from build123d import *

# Parameters (mm, degrees)
F0_W          = 54
F0_H          = 54
F1_DEPTH      = 2
F2_W          = 54
F2_H          = 54
F2_W_2        = 50.3
F2_H_2        = 50.3
F3_DEPTH      = 10.2
F4_R          = 3.5
F5_DEPTH      = 5.5
F6_R          = 1.6
F7_DEPTH      = 25
F8_W          = 9.5
F8_H          = 4.75
F9_DEPTH      = 25
F11_DEPTH     = 25
F12_T1_DEPTH  = 48
F12_T3_DEPTH  = 48
F12_T5_DEPTH  = 16.7
F12_S9_W      = 3
F12_S9_H      = 3
F12_T10_DEPTH = 3
F12_S15_W     = 3
F12_S15_H     = 3
F12_T16_DEPTH = 3
F12_S21_W     = 3
F12_S21_H     = 3
F12_T22_DEPTH = 3
F12_S27_W     = 3
F12_S27_H     = 3
F12_T28_DEPTH = 3
F13_R         = 3
F14_DEPTH     = 2.5
F15_R         = 0.8
F16_R         = 2


# Not quite as in the source:
# - a fillet or chamfer that OpenCascade refuses, or shapes differently, is made with other operations: its cross-section is extruded or revolved along the edge and cut away or added


with BuildPart() as f1:
    # F0 (on Top) → F1 (new body)
    with BuildSketch(Plane.XY):
        Rectangle(F0_W, F0_H)
    extrude(amount=F1_DEPTH)

    # F2 (on face) → F3 (join)
    with BuildSketch(Plane.XY.offset(2)):
        Rectangle(F2_W, F2_H)
        Rectangle(F2_W_2, F2_H_2, mode=Mode.SUBTRACT)
    extrude(amount=F3_DEPTH)

    # F4 (on face) → F5 (join)
    with BuildSketch(Plane.XY.offset(2)):
        with Locations((-22.5, 22.5)):
            Circle(F4_R)
        with Locations((22.5, 22.5)):
            Circle(F4_R)
        with Locations((22.5, -22.5)):
            Circle(F4_R)
        with Locations((-22.5, -22.5)):
            Circle(F4_R)
    extrude(amount=F5_DEPTH)

    # F6 (on face) → F7 (cut)
    with BuildSketch(Plane(origin=(0, 0, 0), x_dir=(1, 0, 0), z_dir=(0, 0, -1))):
        with Locations((-22.5, 22.5)):
            Circle(F6_R)
        with Locations((22.5, 22.5)):
            Circle(F6_R)
        with Locations((22.5, -22.5)):
            Circle(F6_R)
        with Locations((-22.5, -22.5)):
            Circle(F6_R)
        Circle(F6_R)
    extrude(amount=-F7_DEPTH, mode=Mode.SUBTRACT)

    # F8 (on face) → F9 (cut)
    with BuildSketch(Plane.XZ.offset(27)):
        with Locations((13.25, 5.875)):
            Rectangle(F8_W, F8_H)
    extrude(amount=-F9_DEPTH, mode=Mode.SUBTRACT)

    # F10 (on face) → F11 (cut)
    with BuildSketch(Plane.XY.offset(2)):
        with BuildLine():
            add(Edge.make_bspline(
                [(-20.15, 4.5483106502), (-23.5056844979, 4.5483106502), (-21.827842249, -2.2741553251), (-20.15, -9.0966213004), (-18.472157751, -2.2741553251), (-16.7943155021, 4.5483106502), (-20.15, 4.5483106502)],
                knots=[0, 0, 0, 2.0943951024, 2.0943951024, 4.1887902048, 4.1887902048, 6.2831853072, 6.2831853072, 6.2831853072], degree=2, weights=[1, 0.5, 1, 0.5, 1, 0.5, 1]))
        make_face()
    extrude(amount=-F11_DEPTH, mode=Mode.SUBTRACT)

    # F12: fillet of radius 3 on 8 edges, made by hand

    # F12_s2 → F12_t1 (cut)
    with BuildSketch(Plane.YZ.offset(-24)):
        with BuildLine():
            ThreePointArc((-24, 0), (-26.1213203436, 0.8786796564), (-27, 3))
            Line((-27, 3), (-27, 0))
            Line((-27, 0), (-24, 0))
        make_face()
        with BuildLine():
            ThreePointArc((27, 3), (26.1213203436, 0.8786796564), (24, 0))
            Line((24, 0), (27, 0))
            Line((27, 0), (27, 3))
        make_face()
    extrude(amount=F12_T1_DEPTH, mode=Mode.SUBTRACT)

    # F12_s4 → F12_t3 (cut)
    with BuildSketch(Plane.XZ.offset(-24)):
        with BuildLine():
            ThreePointArc((-27, 3), (-26.1213203436, 0.8786796564), (-24, 0))
            Line((-24, 0), (-27, 0))
            Line((-27, 0), (-27, 3))
        make_face()
        with BuildLine():
            ThreePointArc((27, 3), (26.1213203436, 0.8786796564), (24, 0))
            Line((24, 0), (27, 0))
            Line((27, 0), (27, 3))
        make_face()
    extrude(amount=F12_T3_DEPTH, mode=Mode.SUBTRACT)

    # F12_s6 → F12_t5 (cut)
    with BuildSketch(Plane.XY.offset(3)):
        with BuildLine():
            ThreePointArc((27, -24), (26.1213203436, -26.1213203436), (24, -27))
            Line((24, -27), (27, -27))
            Line((27, -27), (27, -24))
        make_face()
        with BuildLine():
            ThreePointArc((-27, -24), (-26.1213203436, -26.1213203436), (-24, -27))
            Line((-24, -27), (-27, -27))
            Line((-27, -27), (-27, -24))
        make_face()
        with BuildLine():
            ThreePointArc((-24, 27), (-26.1213203436, 26.1213203436), (-27, 24))
            Line((-27, 24), (-27, 27))
            Line((-27, 27), (-24, 27))
        make_face()
        with BuildLine():
            ThreePointArc((24, 27), (26.1213203436, 26.1213203436), (27, 24))
            Line((27, 24), (27, 27))
            Line((27, 27), (24, 27))
        make_face()
    extrude(amount=F12_T5_DEPTH, mode=Mode.SUBTRACT)


with BuildPart() as f12_tool8:
    # F12_s9 → F12_t10 (new body)
    with BuildSketch(Plane.YZ.offset(-24)):
        with Locations((-25.5, 1.5)):
            Rectangle(F12_S9_W, F12_S9_H)
    extrude(amount=-F12_T10_DEPTH)

    # F12_s11 → F12_t12 (revolve, cut)
    with BuildSketch(Plane(origin=(-24, -24, 3), x_dir=(0, 0.7071067812, 0.7071067812), z_dir=(0, -0.7071067812, 0.7071067812))):
        with BuildLine():
            ThreePointArc((0, -3), (3, 0), (0, 3))
            Line((0, 3), (0, -3))
        make_face()
    revolve(axis=Axis((-24, -24, 3), (-1, 0, 0)), mode=Mode.SUBTRACT)


with BuildPart() as f1_1:
    add(f1.part)

    # F12_t7: cut F12_tool8
    add(f12_tool8.part, mode=Mode.SUBTRACT)


with BuildPart() as f12_tool14:
    # F12_s15 → F12_t16 (new body)
    with BuildSketch(Plane.YZ.offset(24)):
        with Locations((-25.5, 1.5)):
            Rectangle(F12_S15_W, F12_S15_H)
    extrude(amount=F12_T16_DEPTH)

    # F12_s17 → F12_t18 (revolve, cut)
    with BuildSketch(Plane(origin=(24, -24, 3), x_dir=(0, 0.7071067812, 0.7071067812), z_dir=(0, 0.7071067812, -0.7071067812))):
        with BuildLine():
            ThreePointArc((0, -3), (3, 0), (0, 3))
            Line((0, 3), (0, -3))
        make_face()
    revolve(axis=Axis((24, -24, 3), (1, 0, 0)), mode=Mode.SUBTRACT)


with BuildPart() as f1_2:
    add(f1_1.part)

    # F12_t13: cut F12_tool14
    add(f12_tool14.part, mode=Mode.SUBTRACT)


with BuildPart() as f12_tool20:
    # F12_s21 → F12_t22 (new body)
    with BuildSketch(Plane.XZ.offset(-24)):
        with Locations((-25.5, 1.5)):
            Rectangle(F12_S21_W, F12_S21_H)
    extrude(amount=-F12_T22_DEPTH)

    # F12_s23 → F12_t24 (revolve, cut)
    with BuildSketch(Plane(origin=(-24, 24, 3), x_dir=(0.7071067812, 0, 0.7071067812), z_dir=(-0.7071067812, 0, 0.7071067812))):
        with BuildLine():
            ThreePointArc((0, -3), (3, 0), (0, 3))
            Line((0, 3), (0, -3))
        make_face()
    revolve(axis=Axis((-24, 24, 3), (0, 1, 0)), mode=Mode.SUBTRACT)


with BuildPart() as f1_3:
    add(f1_2.part)

    # F12_t19: cut F12_tool20
    add(f12_tool20.part, mode=Mode.SUBTRACT)


with BuildPart() as f12_tool26:
    # F12_s27 → F12_t28 (new body)
    with BuildSketch(Plane.XZ.offset(-24)):
        with Locations((25.5, 1.5)):
            Rectangle(F12_S27_W, F12_S27_H)
    extrude(amount=-F12_T28_DEPTH)

    # F12_s29 → F12_t30 (revolve, cut)
    with BuildSketch(Plane(origin=(24, 24, 3), x_dir=(-0.7071067812, 0, 0.7071067812), z_dir=(-0.7071067812, 0, -0.7071067812))):
        with BuildLine():
            ThreePointArc((0, -3), (3, 0), (0, 3))
            Line((0, 3), (0, -3))
        make_face()
    revolve(axis=Axis((24, 24, 3), (0, 1, 0)), mode=Mode.SUBTRACT)


with BuildPart() as f1_4:
    add(f1_3.part)

    # F12_t25: cut F12_tool26
    add(f12_tool26.part, mode=Mode.SUBTRACT)

    # F13 (on face) → F14 (cut)
    with BuildSketch(Plane(origin=(0, 0, 0), x_dir=(1, 0, 0), z_dir=(0, 0, -1))):
        with Locations((-22.5, 22.5)):
            Circle(F13_R)
        with Locations((22.5, 22.5)):
            Circle(F13_R)
        with Locations((22.5, -22.5)):
            Circle(F13_R)
        with Locations((-22.5, -22.5)):
            Circle(F13_R)
    extrude(amount=-F14_DEPTH, mode=Mode.SUBTRACT)

    # F15
    f15_edges = [f1_4.edges().sort_by_distance(p)[0] for p in [
        (8.5, -26.075, 8.25),
        (8.5, -26.075, 3.5),
        (18, -26.075, 3.5),
        (18, -26.075, 8.25),
    ]]
    fillet(f15_edges, radius=F15_R)

    # F16
    f16_edges = [f1_4.edges().sort_by_distance(p)[0] for p in [
        (-25.15, 25.15, 7.1),
        (25.15, 25.15, 7.1),
        (-25.15, -25.15, 7.1),
        (25.15, -25.15, 7.1),
    ]]
    fillet(f16_edges, radius=F16_R)


solid = f1_4.part
Geometry: final body of the model. Coordinates: model frame, mm. A direction names the side the tool comes from. Coordinates: 2 decimals unless noted, no trailing zeros. Order: outer loops, then holes, each group sorted by start corner. A loop starts at its lowest first (then second) coordinate and runs counter-clockwise, first axis right, second up.
1) Section B-B (z = 9.75). Return loops of the section in (x, y), then the cut area to 3 significant figures.
Result sheet:
outline: (-27, -24) arc R3 ccw to (-24, -27) - (24, -27) arc R3 ccw to (27, -24) - (27, 24) arc R3 ccw to (24, 27) - (-24, 27) arc R3 ccw to (-27, 24) - close; hole (-25.15, -23.15) arc R2 ccw to (-23.15, -25.15) - (23.15, -25.15) arc R2 ccw to (25.15, -23.15) - (25.15, 23.15) arc R2 ccw to (23.15, 25.15) - (-23.15, 25.15) arc R2 ccw to (-25.15, 23.15) - close
area: 382 mm2
2) Section C-C (y = -13.5). Return loops of the section in (x, z), then the cut area to 3 significant figures.
Result sheet:
outline: (-27, 3) arc R3 ccw to (-24, 0) - (24, 0) arc R3 ccw to (27, 3) - (27, 12.2) - (25.15, 12.2) - (25.15, 2) - (-25.15, 2) - (-25.15, 12.2) - (-27, 12.2) - close
area: 142 mm2
3) First-contact query: P1, Ø3.5, axis at x = -22.5, y = 22.5, coming from the -Z side; P2, Ø2, axis at x = 13, y = -26, coming from the -Z side; P3, Ø6, axis at x = -8.5, y = 16, coming from the +Z side. Flat tips, straight axial feed; report the tip coordinate or a pass-through.
Result sheet:
P1: stops at z = 2.5
P2: stops at z = 0.17
P3: stops at z = 2
4) Section A-A (x = 0). Return loops of the section in (y, z), then the cut area to 3 significant figures.
Result sheet:
outline: (-27, 3) arc R3 ccw to (-24, 0) - (-1.6, 0) - (-1.6, 2) - (-25.15, 2) - (-25.15, 12.2) - (-27, 12.2) - close; (1.6, 0) - (24, 0) arc R3 ccw to (27, 3) - (27, 12.2) - (25.15, 12.2) - (25.15, 2) - (1.6, 2) - close
area: 135 mm2
5) Ray query, probe 1 along Y at (x, z) = (-22.5, 5.35); probe 2 along Y at (x, z) = (12, 9.75). Return the intervals inside material, ascending.
Result sheet:
probe 1: y = -27 to -24.1, -20.9 to -19, 19 to 20.9, 24.1 to 27
probe 2: y = -27 to -25.15, 25.15 to 27
6) Set-up query: faces 4 (the flat face through (8.5, -26, 6)), 5 (the cylindrical face through (20.1, -20.7, 1.2)), 6 (the flat face through (-22.12, 20.75, 7.5)). Return all of +Z, -Z, +X, -X, +Y, -Y with unobstructed straight access to the full face (end or side cutting, diameter ignored); none if empty.
Result sheet:
face 4: -Y
face 5: -Z
face 6: +Z
7) Draft query along X for faces 1 (the cylindrical face through (-26.14, -26.1, 7.54)), 2 (the cylindrical face through (-24.55, -24.58, 9.88)), 3 (the cylindrical face through (26.14, 0.34, 0.9)). Return one class per face: released by +X, released by -X, zero draft, split by the parting line, or undercut.
Result sheet:
face 1: released by -X
face 2: undercut
face 3: released by +X
8) Section D-D (x = 22.5). Return loops of the section in (y, z), then the cut area to 3 significant figures.
Result sheet:
outline: (-27, 3) arc R3 ccw to (-25.5, 0.4) - (-25.5, 2.5) - (-24.1, 2.5) - (-24.1, 7.5) - (-25.15, 7.5) - (-25.15, 12.2) - (-27, 12.2) - close; (-20.9, 2.5) - (-19.5, 2.5) - (-19.5, 0) - (19.5, 0) - (19.5, 2.5) - (20.9, 2.5) - (20.9, 7.5) - (19, 7.5) - (19, 2) - (-19, 2) - (-19, 7.5) - (-20.9, 7.5) - close; (24.1, 2.5) - (25.5, 2.5) - (25.5, 0.4) arc R3 ccw to (27, 3) - (27, 12.2) - (25.15, 12.2) - (25.15, 7.5) - (24.1, 7.5) - close
area: 148 mm2
